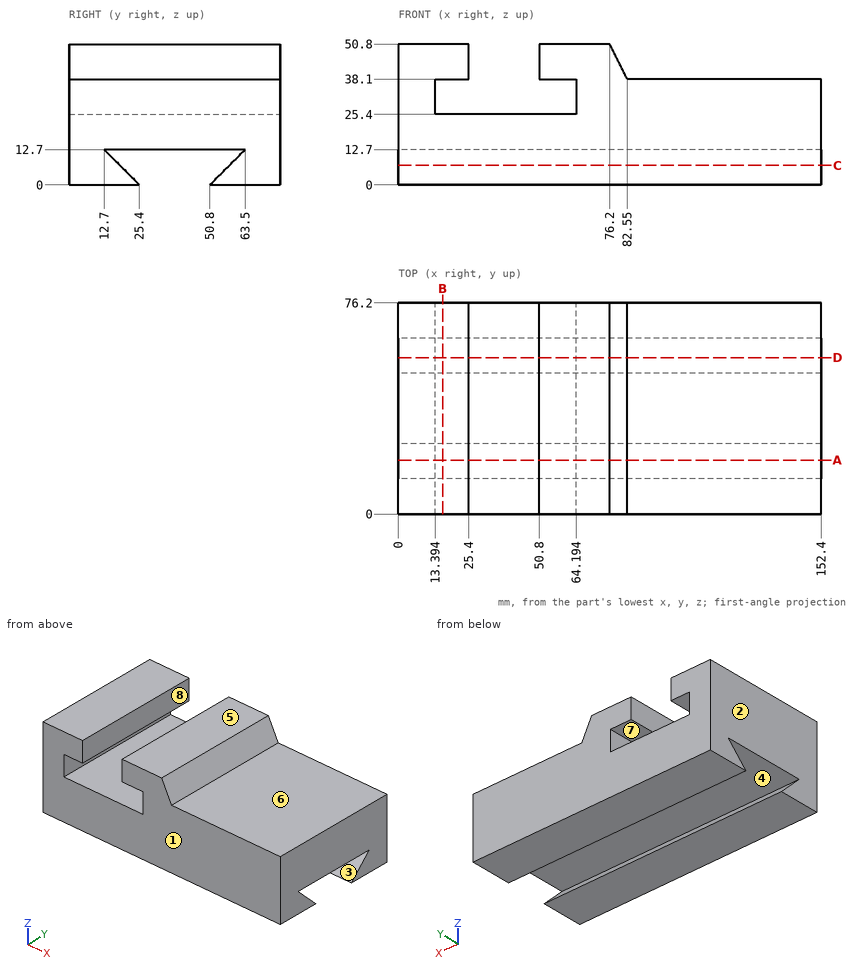
Job drawing, mm, ordinate dimensions from the low corner. One solid piece. A direction names the side the tool comes from. Give positions to 0.01 mm unless a question says otherwise; leave off trailing zeros. Write each loop counter-clockwise with the first axis right and the second up, starting at its lowest first coordinate (ties: lowest second). Pieces come first, ordered by that corner, then holes. Notation, with made-up numbers: M 8,19 L 55,19 A4 cw 55,25 Z; hole C 10,-25 d7. An arc over 180 degrees is marked long. Put each result on its own line as item: value. Start each with the question number.
(1) Mould opens along Y. For the marked faces 1, 2, 3 and 4 say: +Y half, -Y half, draft (parallel to the pull), parting line (faces both ways), or undercut.
(2) Band-saw the part on D-D, the plane y = 56.5. Write the cut outline in (x, z).
(3) Band-saw the part on A-A, the plane y = 19.5. Write the cut outline in (x, z).
(4) Flat gauge pins, fed straight in: pin 1 Ø5 at (y, z) = (33, 44.5) entering from +X; pin 2 Ø1.5 at (x, y) = (48, 66.5) entering from +Z; pin 3 Ø21 at (x, y) = (115.5, 43) entering from +Z; pin 4 Ø14 at (y, z) = (45, 44.5) entering from -X. Where does each tip first touch, or does it go through?
(5) Which spindle directions (+Z, -Z, +X, -X, +Y, -Y) get a long thin tool onto all of the face, cutting with end or side? Do the marked faces 5, 6, 7 and 8. Say none if no direction does.
(6) Probe L1, parallel to X at y = 28, z = 25.5; L2, parallel to Z at x = 61, y = 23.5; L3, parallel to Z at x = 19, y = 38.5. List the from-to ranges inside material, lowest first.
(7) Band-saw the part on B-B, the plane x = 16. Write the cut outline in (y, z), and give its area (3 significant figures).
(8) Band-saw the part on C-C, the plane z = 7. Write the cut outline in (x, y).
Response values:
1. face 1: -Y half
1. face 2: draft
1. face 3: undercut
1. face 4: undercut
2. outline: M 0,0 L 152.4,0 L 152.4,5.7 L 0,5.7 Z; M 0,12.7 L 152.4,12.7 L 152.4,38.1 L 82.55,38.1 L 76.2,50.8 L 50.8,50.8 L 50.8,38.1 L 64.19,38.1 L 64.19,25.4 L 13.39,25.4 L 13.39,38.1 L 25.4,38.1 L 25.4,50.8 L 0,50.8 Z
3. outline: M 0,0 L 152.4,0 L 152.4,5.9 L 0,5.9 Z; M 0,12.7 L 152.4,12.7 L 152.4,38.1 L 82.55,38.1 L 76.2,50.8 L 50.8,50.8 L 50.8,38.1 L 64.19,38.1 L 64.19,25.4 L 13.39,25.4 L 13.39,38.1 L 25.4,38.1 L 25.4,50.8 L 0,50.8 Z
4. pin 1: stops at x = 80.6
4. pin 2: stops at z = 25.4
4. pin 3: stops at z = 38.1
4. pin 4: stops at x = 0
5. face 5: +Z, +X, -X, +Y, -Y
5. face 6: +Z, +X, +Y, -Y
5. face 7: +Y, -Y
5. face 8: +Z, +Y, -Y
6. L1: x = 0 to 13.39, 64.19 to 152.4
6. L2: z = 0 to 1.9, 12.7 to 25.4, 38.1 to 50.8
6. L3: z = 12.7 to 25.4, 38.1 to 50.8
7. outline: M 0,0 L 25.4,0 L 12.7,12.7 L 63.5,12.7 L 50.8,0 L 76.2,0 L 76.2,25.4 L 0,25.4 Z; M 0,38.1 L 76.2,38.1 L 76.2,50.8 L 0,50.8 Z
7. area: 2,420 mm2
8. outline: M 0,0 L 152.4,0 L 152.4,18.4 L 0,18.4 Z; M 0,57.8 L 152.4,57.8 L 152.4,76.2 L 0,76.2 Z
